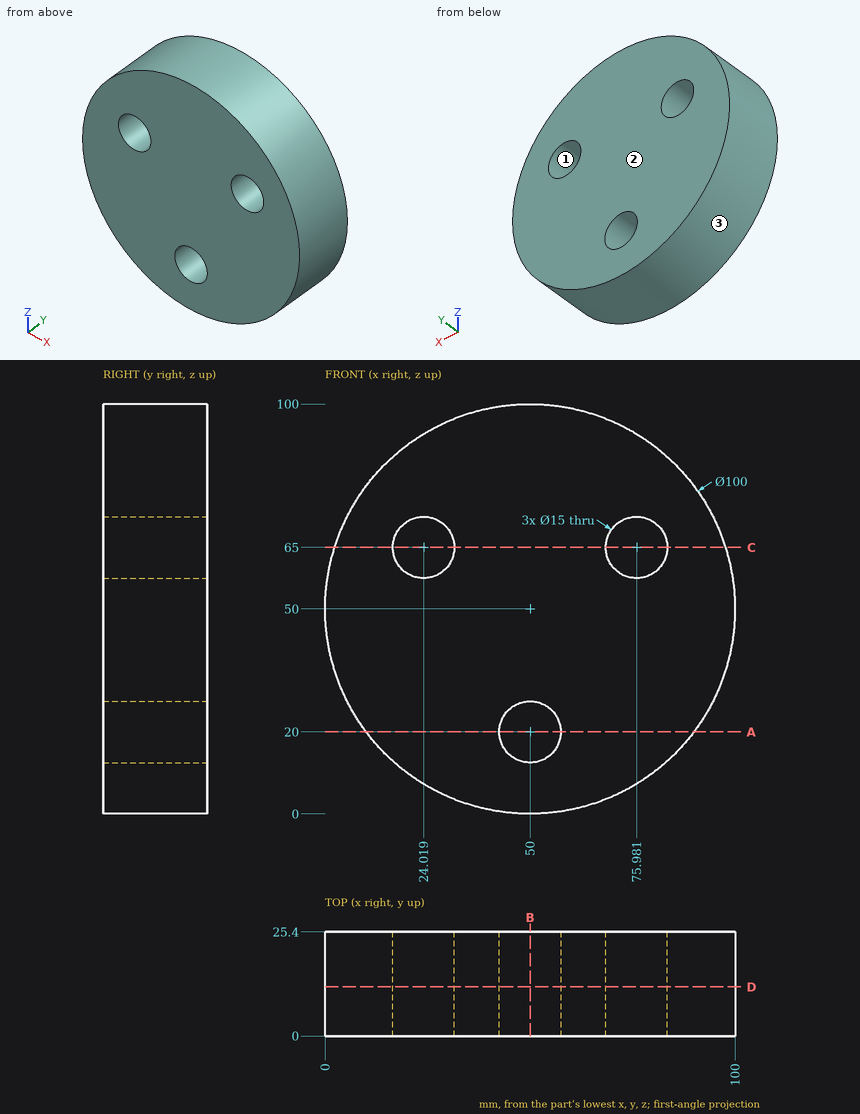
Study the drawing (mm; zero at the part's minimum x, y, z) and answer. Coordinates: 2 decimals unless noted, no trailing zeros. Write each loop counter-clockwise with the first axis right and the second up, starting at its lowest first coordinate (ties: lowest second). Pieces come first, ordered by that corner, then holes. Notation, with made-up numbers: (40, 65.5) - (56, 65.5) arc R25 cw to (56, 101.5) - close; hole circle Ø4 at (78.25, -30.5). An arc over 180 degrees is marked (long way). One line per item, written item: value.
1) Find section B-B (x = 50). Give the vertices of the cut face in (y, z), and give its area (3 significant figures).
Geometry check:
outline: (0, 0) - (25.4, 0) - (25.4, 12.5) - (0, 12.5) - close; (0, 27.5) - (25.4, 27.5) - (25.4, 100) - (0, 100) - close
area: 2,160 mm2
2) Each of these flat-tipped pins is pushed along its axis until it touches: pin 1 Ø2 at (x, y) = (26.5, 6) entering from -Z; pin 2 Ø8 at (x, y) = (17, 11.5) entering from +Z; pin 3 Ø2 at (y, z) = (13, 23.5) entering from +X. Where does it stop, or does it pass through?
Geometry check:
pin 1: stops at z = 5.35
pin 2: stops at z = 90.73
pin 3: stops at x = 93.01
3) Find section C-C (z = 65). Give the vertices of the cut face in (x, y), and give its area (3 significant figures).
Geometry check:
outline: (2.3, 0) - (16.52, 0) - (16.52, 25.4) - (2.3, 25.4) - close; (31.52, 0) - (68.48, 0) - (68.48, 25.4) - (31.52, 25.4) - close; (83.48, 0) - (97.7, 0) - (97.7, 25.4) - (83.48, 25.4) - close
area: 1,660 mm2
4) For a pull along Z with two mould halves and no side action, classify the marked faces 1, 2 and 3 as pulls with the +Z half, pulls with the -Z half, needs draft (parallel to the pull), parting line crosses it, or undercut.
Geometry check:
face 1: undercut
face 2: needs draft
face 3: parting line crosses it
5) Find section D-D (y = 12). Give the vertices of the cut face in (x, z) (1 decimal), and give its area (3 significant figures).
Geometry check:
outline: circle Ø100 at (50, 50); hole circle Ø15 at (24, 65); hole circle Ø15 at (50, 20); hole circle Ø15 at (76, 65)
area: 7,320 mm2
6) Consider line 1 along Z through (x, y) = (50, 16.5); line 2 along X through (y, z) = (19, 71.5); line 3 along X through (y, z) = (16.25, 20). Determine where each line is inside the solid, lowest interval first. Write a range as from..to.
Geometry check:
line 1: z = 0..12.5, 27.5..100
line 2: x = 4.86..20.28, 27.76..72.24, 79.72..95.14
line 3: x = 10..42.5, 57.5..90
7) Find section A-A (z = 20). Give the vertices of the cut face in (x, y), and give its area (3 significant figures).
Geometry check:
outline: (10, 0) - (42.5, 0) - (42.5, 25.4) - (10, 25.4) - close; (57.5, 0) - (90, 0) - (90, 25.4) - (57.5, 25.4) - close
area: 1,650 mm2
